For this review, take the finished solid that the model builds, in its own axes (mm). A direction names the side the tool comes from. Give positions to 0.01 mm unless a question says otherwise; leave off trailing zeros. Write each loop counter-clockwise with the first axis right and the second up, starting at its lowest first coordinate (ties: lowest second). Pieces come first, ordered by that corner, then holes. Notation, with made-up numbers: (-12, 53) -> (43, 53) arc R18 ccw to (43, 79) -> close; hole circle Ø11 at (0, 17.5). An arc over 180 degrees is marked (long way). Return JSON: item names as keys, results as strings.
Autodesk Inventor part; units mm, degrees
ref_plane "YZ Plane" through (0, 0, 0) normal (1, 0, 0) x (0, 1, 0)
ref_plane "XZ Plane" through (0, 0, 0) normal (0, 1, 0) x (-1, 0, 0)
ref_plane "XY Plane" through (0, 0, 0) normal (0, 0, 1) x (1, 0, 0)
sketch "Sketch1" plane through (0, 0, 0) normal (0, 1, 0) x (-1, 0, 0)
  line L0 (-3, 0) -> (-82, 0)
  line L1 (-85, -3) -> (-85, -53)
  line L2 (-82, -56) -> (-3, -56)
  line L3 (0, -53) -> (0, -3)
  arc A0 (-3, -56) -> (0, -53) centre (-3, -53) ccw
  arc A1 (0, -3) -> (-3, 0) centre (-3, -3) ccw
  arc A2 (-82, 0) -> (-85, -3) centre (-82, -3) ccw
  arc A3 (-85, -53) -> (-82, -56) centre (-82, -53) ccw
  circle A4 centre (-3.5, -52.5) radius 1.35
  circle A5 centre (-3.5, -3.5) radius 1.35
  circle A6 centre (-61.5, -52.5) radius 1.35
  circle A7 centre (-61.5, -3.5) radius 1.35
  point P0 (0, 0)
  point P1 (-85, -56)
  point P2 (-85, 0)
  point P3 (0, -56)
  dimension "d0" = 85
  dimension "d1" = 56
  dimension "d2" = 3
  dimension "d9" = 2.7
  dimension "d10" = 2.7
  dimension "d15" = 2.7
  dimension "d16" = 2.7
  dimension "d140" = 58
  dimension "d141" = 58
  dimension "d142" = 49
  dimension "d143" = 3.5
extrude "Extrusion1" add sketch "Sketch1" along normal blind 1.5
sketch "Sketch12" plane through (0, 0, 0) normal (0, -1, 0) x (1, 0, 0)
  line L0 (5, -9.5) -> (75.5, -9.5)
  line L1 (75.5, -9.5) -> (75.5, -46.5)
  line L2 (75.5, -46.5) -> (5, -46.5)
  line L3 (5, -46.5) -> (5, -9.5)
  line L4 (82, -56) -> (3, -56)
  line L5 (85, -3) -> (85, -53)
  line L6 (3, 0) -> (82, 0)
  line L7 (0, -53) -> (0, -3)
  point P0 (0, 0)
  dimension "d152" = 9.5
  dimension "d153" = 9.5
  dimension "d154" = 9.5
  dimension "d155" = 5
extrude "Extrusion12" add sketch "Sketch12" along normal blind 12.25
sketch "Sketch13" plane through (0, 0, 0) normal (0, -1, 0) x (1, 0, 0)
  line L0 (10.5, -53.65) -> (16.35, -53.65)
  line L1 (16.35, -53.65) -> (16.35, -48.8)
  line L2 (16.35, -48.8) -> (10.5, -48.8)
  line L3 (10.5, -48.8) -> (10.5, -53.65)
  line L4 (0, -53) -> (0, -3)
  line L5 (82, -56) -> (3, -56)
  point P0 (0, 0)
  dimension "d146" = 10.5
  dimension "d147" = 2.35
  dimension "d148" = 4.85
  dimension "d149" = 5.85
extrude "Extrusion13" cut sketch "Sketch13" against normal up to next
properties part number "Pi4BatteryBoard_Mockup"
1. Add section B-B, the plane z = -41. State the section outline as (x, y) points, plus the area to 3 significant figures.
Results found:
{"outline": "(0, 0) -> (5, 0) -> (5, -12.25) -> (75.5, -12.25) -> (75.5, 0) -> (85, 0) -> (85, 1.5) -> (0, 1.5) -> close", "area": "991 mm²"}
2. To check wall thickness, follow probe 1 along Z at (x, y) = (61.5, 0.95); probe 2 along Y at (x, z) = (14, -8); probe 3 along X at (y, z) = (-11.5, -21.5). State the ranges of each line that lie inside material, in increasing order.
Results found:
{"probe 1": "z = -56 to -53.85, -51.15 to -4.85, -2.15 to 0", "probe 2": "y = 0 to 1.5", "probe 3": "x = 5 to 75.5"}
3. Add section A-A, the plane x = 61.5. State the section outline as (y, z) points.
Results found:
{"outline": "(-12.25, -46.5) -> (0, -46.5) -> (0, -51.15) -> (1.5, -51.15) -> (1.5, -4.85) -> (0, -4.85) -> (0, -9.5) -> (-12.25, -9.5) -> close; (0, -56) -> (1.5, -56) -> (1.5, -53.85) -> (0, -53.85) -> close; (0, -2.15) -> (1.5, -2.15) -> (1.5, 0) -> (0, 0) -> close"}
4. For pin 1 (3 mm diameter, centred on x = 61.5, z = -52.5, fed in from -Y); pin 2 (3 mm diameter, centred on x = 57.5, y = -4, fed in from +Z); pin 3 (6 mm diameter, centred on x = 25, y = -7, fed in from -Z), all flat-tipped, find the tip position at first contact; note any pin that passes through.
Results found:
{"pin 1": "stops at y = 0", "pin 2": "stops at z = -9.5", "pin 3": "stops at z = -46.5"}
5. Add section D-D, the plane z = -8. State the section outline as (x, y) points, plus the area to 4 significant figures.
Results found:
{"outline": "(0, 0) -> (85, 0) -> (85, 1.5) -> (0, 1.5) -> close", "area": "127.5 mm²"}
6. The part is to be moulded in two halves that separate along X. For faces 5 (the flat face through (5, -6, -28)), 6 (the flat face through (53, 0, -9)), 7 (the cylindrical face through (3.79, 0.74, -51.18)), 8 (the cylindrical face through (61.79, 0.74, -2.18)), say which applies: +X half, -X half, draft (parallel to the pull), parting line (faces both ways), or undercut.
Results found:
{"face 5": "-X half", "face 6": "draft", "face 7": "undercut", "face 8": "undercut"}
7. For faces 1 (the flat face through (75.5, -6, -28)), 2 (the cylindrical face through (84.14, 0.74, -0.9)), 3 (the flat face through (41, -6, -46.5)), 4 (the flat face through (40, -6, -9.5)), list the 3-axis set-ups (+Z, -Z, +X, -X, +Y, -Y) from which the entire face can be reached by the end or side of a thin tool; tool diameter is ignored.
Results found:
{"face 1": "+Z, -Z, +X, -Y", "face 2": "+Z, +X, +Y, -Y", "face 3": "-Z, +X, -X, -Y", "face 4": "+Z, +X, -X, -Y"}
8. Add section C-C, the plane y = -7.5. State the section outline as (x, z) points.
Results found:
{"outline": "(5, -46.5) -> (75.5, -46.5) -> (75.5, -9.5) -> (5, -9.5) -> close"}
